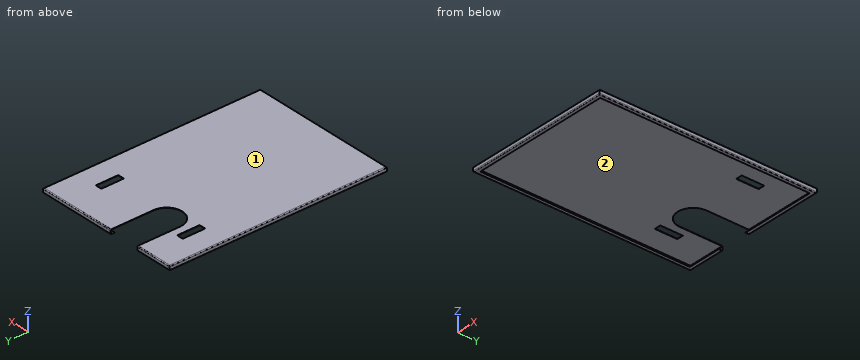
from build123d import *

# Parameters (mm, degrees)
SKETCH_1_W          = 568
SKETCH_1_H          = 839
SKETCH_1_W_2        = 25
SKETCH_1_H_2        = 87
EXTRUDE_1_DEPTH     = 1.2
SKETCH_2_W          = 568
SKETCH_2_H          = 839
SKETCH_2_W_2        = 565.6
SKETCH_2_H_2        = 836.6
EXTRUDE_2_DEPTH     = 15.5
SKETCH_3_W          = 568
SKETCH_3_H          = 839
SKETCH_3_W_2        = 538
SKETCH_3_H_2        = 809
EXTRUDE_3_DEPTH     = 1.2
FILLET_1_R          = 2
FILLET_2_R          = 3.2
FILLET_3_R          = 3.2
CUT_EXTRUDE_1_DEPTH = 1014.323191287


with BuildPart() as part:
    # 스케치1 → 보스-돌출1 (new body)
    with BuildSketch(Plane.XY):
        with Locations((284, 419.5)):
            Rectangle(SKETCH_1_W, SKETCH_1_H)
        with Locations((101.5, 668.5)):
            Rectangle(SKETCH_1_W_2, SKETCH_1_H_2, mode=Mode.SUBTRACT)
        with Locations((466.5, 668.5)):
            Rectangle(SKETCH_1_W_2, SKETCH_1_H_2, mode=Mode.SUBTRACT)
    extrude(amount=EXTRUDE_1_DEPTH)

    # 스케치2 → 보스-돌출2 (add)
    with BuildSketch(Plane(origin=(0, 0, 0), x_dir=(-1, 0, 0), z_dir=(0, 0, -1))):
        with Locations((-284, 419.5)):
            Rectangle(SKETCH_2_W, SKETCH_2_H)
        with Locations((-284, 419.5)):
            Rectangle(SKETCH_2_W_2, SKETCH_2_H_2, mode=Mode.SUBTRACT)
    extrude(amount=EXTRUDE_2_DEPTH)

    # 스케치3 → 보스-돌출3 (add)
    with BuildSketch(Plane(origin=(0, 0, -15.5), x_dir=(-1, 0, 0), z_dir=(0, 0, -1))):
        with Locations((-284, 419.5)):
            Rectangle(SKETCH_3_W, SKETCH_3_H)
        with Locations((-284, 419.5)):
            Rectangle(SKETCH_3_W_2, SKETCH_3_H_2, mode=Mode.SUBTRACT)
    extrude(amount=-EXTRUDE_3_DEPTH)

    # 필렛1
    fillet_1_edges = [part.edges().sort_by_distance(p)[0] for p in [
        (1.2, 419.5, 0),
        (284, 837.8, 0),
        (566.8, 419.5, 0),
        (284, 1.2, 0),
        (566.8, 1.2, -7.15),
        (1.2, 1.2, -7.15),
        (284, 1.2, -14.3),
        (566.8, 837.8, -7.15),
        (1.2, 837.8, -7.15),
        (1.2, 419.5, -14.3),
        (284, 837.8, -14.3),
        (566.8, 419.5, -14.3),
    ]]
    fillet(fillet_1_edges, radius=FILLET_1_R)

    # 필렛2
    fillet_2_edges = [part.edges().sort_by_distance(p)[0] for p in [
        (568, 419.5, 1.2),
        (284, 839, 1.2),
        (0, 419.5, 1.2),
        (284, 0, 1.2),
    ]]
    fillet(fillet_2_edges, radius=FILLET_2_R)

    # 필렛3
    fillet_3_edges = [part.edges().sort_by_distance(p)[0] for p in [
        (284, 0, -15.5),
        (0, 419.5, -15.5),
        (284, 839, -15.5),
        (568, 419.5, -15.5),
    ]]
    fillet(fillet_3_edges, radius=FILLET_3_R)

    # 스케치4 → 컷-돌출1 (cut, through all)
    with BuildSketch(Plane.XY.offset(1.2)):
        with BuildLine():
            Line((265, 952.257222416), (265, 674))
            ThreePointArc((265, 674), (205, 614), (145, 674))
            Line((145, 674), (145, 952.257222416))
            ThreePointArc((145, 952.257222416), (205, 1012.257222416), (265, 952.257222416))
        make_face()
    extrude(amount=-CUT_EXTRUDE_1_DEPTH, mode=Mode.SUBTRACT)


solid = part.part
For this review, take the finished solid that the model builds, in its own axes (mm). Face numbers are marked on the shaded views. Round coordinates to 2 decimals unless told otherwise and drop trailing zeros. Order: outer loops, then holes, each group sorted by start corner. A loop starts at its lowest first (then second) coordinate and runs counter-clockwise, first axis right, second up. Notation, with made-up numbers: (38.5, -31.5) -> (59.5, -31.5) arc R17 cw to (59.5, 0.5) -> close; hole circle Ø1 at (39.5, 11.25). An arc over 180 degrees is marked (long way). Write item = value, one per line. Start each with the question number.
1) The part is to be moulded in two halves that separate along X. For the marked faces 1 and 2, say which applies: +X half, -X half, draft (parallel to the pull), parting line (faces both ways), or undercut.
2) Take a section at C-C on z = -5.5. State the section outline as (x, y) points.
3) To check wall thickness, follow line 1 (X direction, y = 593, z = -9.75); line 2 (Y direction, x = 114, z = -8.5); line 3 (Y direction, x = 184.5, z = -4.25). State the ranges of each line that lie inside material, in increasing order. Write a range as from..to.
4) Take a section at D-D on x = 279.5. State the section outline as (y, z) points, plus the area to 3 significant figures.
5) Take a section at A-A on y = 407. State the section outline as (x, z) points.
6) Insertion check: pin 1 (1 mm diameter, centred on y = 230.5, z = -15, fed in from +X); pin 2 (4 mm diameter, centred on x = 172, z = -2.5, fed in from +Y); pin 3 (3 mm diameter, centred on x = 119, y = 247, fed in from -Z). Each pin has a flat end and moves straight along its axis. Give the tip position at first contact, or say it passes through.
7) Take a section at B-B on x = 205. State the section outline as (y, z) points, plus the area to 3 significant figures.
Verdict:
q1.face_1 = draft
q1.face_2 = undercut
q2.outline = (0, 0) -> (568, 0) -> (568, 839) -> (265, 839) -> (265, 837.8) -> (564.8, 837.8) arc R2 cw to (566.8, 835.8) -> (566.8, 3.2) arc R2 cw to (564.8, 1.2) -> (3.2, 1.2) arc R2 cw to (1.2, 3.2) -> (1.2, 835.8) arc R2 cw to (3.2, 837.8) -> (145, 837.8) -> (145, 839) -> (0, 839) -> close
q3.line_1 = 0..1.2, 566.8..568
q3.line_2 = 0..1.2, 837.8..839
q3.line_3 = 0..1.2
q4.outline = (0, -12.3) arc R3.2 ccw to (3.2, -15.5) -> (15, -15.5) -> (15, -14.3) -> (3.2, -14.3) arc R2 cw to (1.2, -12.3) -> (1.2, -2) arc R2 cw to (3.2, 0) -> (835.8, 0) arc R2 cw to (837.8, -2) -> (837.8, -12.3) arc R2 cw to (835.8, -14.3) -> (824, -14.3) -> (824, -15.5) -> (835.8, -15.5) arc R3.2 ccw to (839, -12.3) -> (839, -2) arc R3.2 ccw to (835.8, 1.2) -> (3.2, 1.2) arc R3.2 ccw to (0, -2) -> close
q4.area = 1,070 mm2
q5.outline = (0, -12.3) arc R3.2 ccw to (3.2, -15.5) -> (15, -15.5) -> (15, -14.3) -> (3.2, -14.3) arc R2 cw to (1.2, -12.3) -> (1.2, -2) arc R2 cw to (3.2, 0) -> (564.8, 0) arc R2 cw to (566.8, -2) -> (566.8, -12.3) arc R2 cw to (564.8, -14.3) -> (553, -14.3) -> (553, -15.5) -> (564.8, -15.5) arc R3.2 ccw to (568, -12.3) -> (568, -2) arc R3.2 ccw to (564.8, 1.2) -> (3.2, 1.2) arc R3.2 ccw to (0, -2) -> close
q6.pin_1 = 567.12
q6.pin_2 = 1.88
q6.pin_3 = 0
q7.outline = (0, -12.3) arc R3.2 ccw to (3.2, -15.5) -> (15, -15.5) -> (15, -14.3) -> (3.2, -14.3) arc R2 cw to (1.2, -12.3) -> (1.2, -2) arc R2 cw to (3.2, 0) -> (614, 0) -> (614, 1.2) -> (3.2, 1.2) arc R3.2 ccw to (0, -2) -> close
q7.area = 769 mm2
